Geometry: final body of the model. Coordinates: model frame, mm. A direction names the side the tool comes from. Give positions to 0.01 mm unless a question says otherwise; leave off trailing zeros. Loops run counter-clockwise (first coordinate to the right, second up) from the corner with the lowest first, then second, coordinate; pieces in that order, holes last.
from build123d import *

# Parameters (mm, degrees)
SKETCH1_W           = 12.7
SKETCH1_H           = 119.38
BOSS_EXTRUDE1_DEPTH = 190.5
SKETCH2_W           = 38.1
SKETCH2_H           = 38.1
CUT_EXTRUDE1_DEPTH  = 226.173542851
SKETCH3_W           = 12.7
SKETCH3_H           = 15.677565112
BOSS_EXTRUDE2_DEPTH = 20.9926
SKETCH4_W           = 15.677565112
SKETCH4_H           = 3.864411614
BOSS_EXTRUDE3_DEPTH = 38.1


with BuildPart() as part:
    # Sketch1 → Boss-Extrude1 (new body)
    with BuildSketch(Plane.XY):
        with Locations((-11.213311432, 59.69)):
            Rectangle(SKETCH1_W, SKETCH1_H)
    extrude(amount=BOSS_EXTRUDE1_DEPTH)

    # Sketch2 → Cut-Extrude1 (cut, through all)
    with BuildSketch(Plane.ZY.offset(17.563311432)):
        with Locations((171.45, 19.05)):
            Rectangle(SKETCH2_W, SKETCH2_H)
        with Locations((19.05, 19.05)):
            Rectangle(SKETCH2_W, SKETCH2_H)
    extrude(amount=-CUT_EXTRUDE1_DEPTH, mode=Mode.SUBTRACT)

    # Sketch3 → Boss-Extrude2 (add)
    with BuildSketch(Plane.XZ):
        with Locations((-11.213311432, 107.097101601)):
            Rectangle(SKETCH3_W, SKETCH3_H)
    extrude(amount=BOSS_EXTRUDE2_DEPTH)

    # Sketch4 → Boss-Extrude3 (add)
    with BuildSketch(Plane.ZY.offset(17.563311432)):
        with Locations((107.097101601, -19.060394193)):
            Rectangle(SKETCH4_W, SKETCH4_H)
    extrude(amount=BOSS_EXTRUDE3_DEPTH)


solid = part.part
Item 1: Section query B-B on z = 107.5. Return loops of the section in (x, y).
Values follow:
outline: (-55.66, -20.99) - (-4.86, -20.99) - (-4.86, 119.38) - (-17.56, 119.38) - (-17.56, -17.13) - (-55.66, -17.13) - close
Item 2: Section query C-C on y = 35. Return loops of the section in (x, z), plus the area to 3 significant figures.
Values follow:
outline: (-17.56, 38.1) - (-4.86, 38.1) - (-4.86, 152.4) - (-17.56, 152.4) - close
area: 1,450 mm2
Item 3: Section query D-D on z = 12. Return loops of the section in (x, y).
Values follow:
outline: (-17.56, 38.1) - (-4.86, 38.1) - (-4.86, 119.38) - (-17.56, 119.38) - close
Item 4: Ray query, probe 1 along X at (y, z) = (-9, 105.5); probe 2 along Y at (x, z) = (-15, 91.5); probe 3 along Y at (x, z) = (-13, 180.5). Return the intervals inside material, ascending.
Values follow:
probe 1: x = -17.56 to -4.86
probe 2: y = 0 to 119.38
probe 3: y = 38.1 to 119.38
Item 5: Set-up query: faces 1 (the face through (-55.663, -19, 107)), 2 (the face through (-11, 79, 0)), 3 (the face through (-11, 38.1, 19)), 4 (the face through (-11, 19, 152.4)), 5 (the face through (-36, -17.128, 107)). Return all of +Z, -Z, +X, -X, +Y, -Y with unobstructed straight access to the full face (end or side cutting, diameter ignored); none if empty.
Values follow:
face 1: +Z, -Z, -X, +Y, -Y
face 2: -Z, +X, -X, +Y, -Y
face 3: -Z, +X, -X, -Y
face 4: +Z, +X, -X, -Y
face 5: +Z, -Z, -X, +Y
Item 6: Section query A-A on x = -8. Return loops of the section in (y, z), plus the area to 3 significant figures.
Values follow:
outline: (-20.99, 99.26) - (0, 99.26) - (0, 38.1) - (38.1, 38.1) - (38.1, 0) - (119.38, 0) - (119.38, 190.5) - (38.1, 190.5) - (38.1, 152.4) - (0, 152.4) - (0, 114.94) - (-20.99, 114.94) - close
area: 20,200 mm2
Item 7: Pin query (flat end, axial travel): pin 1 (8 mm diameter, centred on x = -33, z = 104.5, fed in from +Y); pin 2 (4 mm diameter, centred on x = -14.5, z = 129, fed in from -Y); pin 3 (17 mm diameter, centred on x = -20, y = -13, fed in from +Z). Return the tip coordinate at first contact, or that it passes through.
Values follow:
pin 1: stops at y = -17.13
pin 2: stops at y = 0
pin 3: stops at z = 114.94
